The model under review builds one solid part; all positions refer to its coordinate system, in mm. Face numbers are marked on the shaded views. A direction names the side the tool comes from. Give positions to 0.01 mm unless a question says otherwise; leave off trailing zeros. Order: outer loops, then holes, each group sorted by start corner. A loop starts at its lowest first (then second) coordinate and runs counter-clockwise, first axis right, second up.
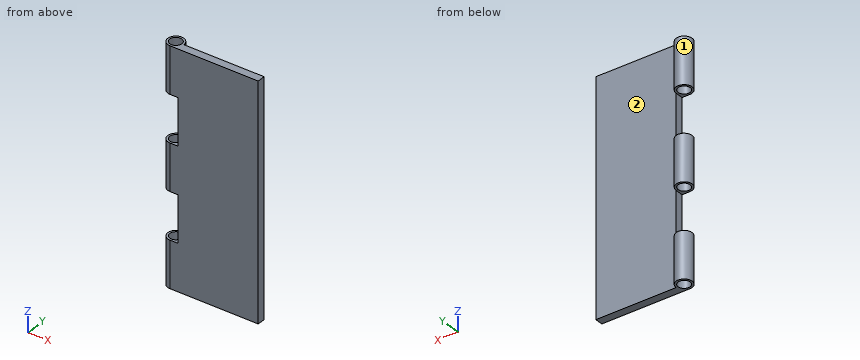
Autodesk Inventor part; units mm, degrees
ref_plane "YZ Plane" through (0, 0, 0) normal (1, 0, 0) x (0, 1, 0)
ref_plane "XZ Plane" through (0, 0, 0) normal (0, 1, 0) x (-1, 0, 0)
ref_plane "XY Plane" through (0, 0, 0) normal (0, 0, 1) x (1, 0, 0)
sketch "Sketch1" plane through (0, 0, 0) normal (0, 0, 1) x (1, 0, 0)
  line L0 (0, 0) -> (-20, 0)
  line L1 (-20, 0) -> (-20, 2)
  line L2 (-20, 2) -> (0, 2)
  line L3 (0, 2) -> (0, 0)
  line L4 (-20, 2) -> (-22, 2)
  line L5 (-22, 2) -> (-22, 4)
  circle A0 centre (-22, 2) radius 2
  line L6 (-22, 0) -> (-20, 0)
  dimension "d0" = 20
  dimension "d1" = 2
  dimension "d2" = 2
  dimension "d3" = 2
extrude "Extrusion1" add sketch "Sketch1" along normal blind 58
sketch "Sketch2" plane through (-20, 2, 0) normal (0, 1, 0) x (1, 0, 0)
  line L0 (0, 0) -> (-2, 0)
  line L1 (-2, 0) -> (-2, -58)
  line L2 (0, -58) -> (-2, -58)
  line L3 (0, 0) -> (0, -58)
  line L4 (20, 0) -> (0, 0)
  line L5 (0, 0) -> (0, -58)
  line L6 (20, -58) -> (0, -58)
  line L7 (20, 0) -> (20, -58)
  line L8 (-4, -58) -> (0, -58)
  line L9 (-4, -58) -> (0, -58)
  line L10 (0, -58) -> (0, -46.4)
  line L11 (0, -46.4) -> (-4, -46.4)
  line L12 (-4, -46.4) -> (-4, -58)
  line L13 (-4, -46.4) -> (0, -46.4)
  line L14 (0, -46.4) -> (0, -34.8)
  line L15 (0, -34.8) -> (-4, -34.8)
  line L16 (-4, -34.8) -> (-4, -46.4)
  line L17 (-4, 0) -> (-4, -58)
  line L18 (0, -34.8) -> (-4, -34.8)
  line L19 (-4, -34.8) -> (-4, -23.2)
  line L20 (-4, -23.2) -> (0, -23.2)
  line L21 (0, -23.2) -> (0, -34.8)
  line L22 (-4, -23.2) -> (0, -23.2)
  line L23 (0, -23.2) -> (0, -11.6)
  line L24 (0, -11.6) -> (-4, -11.6)
  line L25 (-4, -11.6) -> (-4, -23.2)
  line L26 (0, -11.6) -> (-4, -11.6)
  line L27 (-4, -11.6) -> (-4, 0)
  line L28 (-4, 0) -> (0, 0)
  line L29 (0, 0) -> (0, -11.6)
  point P0 (0, -11.6)
  point P1 (-4, -11.6)
  point P2 (0, -23.2)
  dimension "d6" = 11.6
  dimension "d7" = 11.6
  dimension "d8" = 11.6
  dimension "d9" = 11.6
extrude "Extrusion2" cut sketch "Sketch2" along normal mid plane 4 contours L3 L20 L1 L24 | L1 L20 L17 L24 | L3 L11 L1 L15 | L1 L11 L16 L15
sketch "Sketch3" plane through (0, 0, 58) normal (0, 0, 1) x (1, 0, 0)
  line L0 (-22, 0) -> (0, 0)
  line L1 (0, 0) -> (0, 2)
  line L2 (0, 2) -> (-20, 2)
  arc A0 (-20, 2) -> (-22, 0) centre (-22, 2) ccw
hole "Hole1" at (-22, 2, 58) direction (0, 0, -1) diameter 3 end through all
properties part number "SchnierTeilA_CPY"
1. To check wall thickness, follow line 1 (Y direction, x = -22, z = 28); line 2 (X direction, y = 0.8, z = 36); line 3 (Y direction, x = -1.75, z = 52). State the ranges of each line that lie inside material, in increasing order.
2. Take a section at B-B (y = 2.9). Write out the cut boundary in (x, z), and give its area (3 significant figures).
3. Take a section at D-D (z = 21). Write out the cut boundary in (x, y).
4. Insertion check: pin 1 (1 mm diameter, centred on y = 1, z = 38, fed in from -X); pin 2 (4 mm diameter, centred on x = -3.5, z = 12.5, fed in from +Y). Each pin has a flat end and moves straight along its axis. Give the tip position at first contact, or say it passes through.
5. Take a section at C-C (x = -1.5). Write out the cut boundary in (y, z), and give its area (3 significant figures).
6. For the marked faces 1 and 2, list the 3-axis set-ups (+Z, -Z, +X, -X, +Y, -Y) from which the entire face can be reached by the end or side of a thin tool; tool diameter is ignored.
7. Take a section at A-A (z = 49.5). Write out the cut boundary in (x, y).
Answer:
1. line 1: y = 0 to 0.5, 3.5 to 4
1. line 2: x = -20 to 0
1. line 3: y = 0 to 2
2. outline: (-23.79, 0) - (-23.2, 0) - (-23.2, 11.6) - (-23.79, 11.6) - close; (-23.79, 23.2) - (-23.2, 23.2) - (-23.2, 34.8) - (-23.79, 34.8) - close; (-23.79, 46.4) - (-23.2, 46.4) - (-23.2, 58) - (-23.79, 58) - close; (-20.8, 0) - (-20.21, 0) - (-20.21, 11.6) - (-20.8, 11.6) - close; (-20.8, 23.2) - (-20.21, 23.2) - (-20.21, 34.8) - (-20.8, 34.8) - close; (-20.8, 46.4) - (-20.21, 46.4) - (-20.21, 58) - (-20.8, 58) - close
2. area: 40.8 mm2
3. outline: (-20, 0) - (0, 0) - (0, 2) - (-20, 2) - close
4. pin 1: stops at x = -20
4. pin 2: stops at y = 2
5. outline: (0, 0) - (2, 0) - (2, 58) - (0, 58) - close
5. area: 116 mm2
6. face 1: +Z, -Z
6. face 2: +Z, -Z, +X, +Y
7. outline: (-22, 0) - (0, 0) - (0, 2) - (-20, 2) arc R2 ccw (long way) to start; hole circle Ø3 at (-22, 2)
